Design review of the part built by this model. Coordinates are the model's own, in mm. Face numbers are marked on the shaded views. A direction names the side the tool comes from. Round coordinates to 2 decimals unless told otherwise and drop trailing zeros. Loops run counter-clockwise (first coordinate to the right, second up) from the corner with the lowest first, then second, coordinate; pieces in that order, holes last. Notation, with made-up numbers: (88.5, 50.25) - (124.5, 50.25) arc R27 cw to (124.5, 87.25) - close; hole circle Ø2 at (26.25, -24). An arc over 180 degrees is marked (long way). Return JSON: item names as keys, results as strings. Group by question number.
(1) We need section D-D, the plane z = -5.5. Write out the cut boundary in (x, y), and give its area (3 significant figures).
(2) We need section B-B, the plane y = 75. Write out the cut boundary in (x, z) (3 decimals).
(3) We need section C-C, the plane y = 45.5. Write out the cut boundary in (x, z).
(4) We need section A-A, the plane y = 7. Write out the cut boundary in (x, z), and give its area (3 significant figures).
(5) Wall thickness on L1, parallel to Z at x = 18.7, y = 75 (3 decimals); L2, parallel to Y at x = 17, z = -60.5; L3, parallel to Y at x = 10, z = -48.2: over which ranges is each line inside the solid? List them lowest first. Write a range as [from, to].
(6) Clearance check with flat-ended pins moving along their axes: pin 1 (4.5 mm diameter, centred on x = 10, y = -7, fed in from -Z); pin 2 (2 mm diameter, centred on y = 85, z = 1.175, fed in from -X); pin 3 (10 mm diameter, centred on x = 10.5, z = -7.5, fed in from -Y); pin 4 (6 mm diameter, centred on x = 11.5, y = 5, fed in from +Z). State where each tip first meets the part, or that it passes through.
(7) The part is to be moulded in two halves that separate along Z. For the marked faces 1, 2, 3 and 4, say which applies: pulls with the +Z half, pulls with the -Z half, needs draft (parallel to the pull), parting line crosses it, or undercut.
(8) For the marked faces 5, 6, 7, 8 and 9, list the 3-axis set-ups (+Z, -Z, +X, -X, +Y, -Y) from which the entire face can be reached by the end or side of a thin tool; tool diameter is ignored.
from build123d import *

# Parameters (mm, degrees)
EXTRUDE_1_DEPTH     = 2
SKETCH_2_R          = 1.65
CUT_EXTRUDE_1_DEPTH = 2
SKETCH_3_W          = 20
SKETCH_3_H          = 2
EXTRUDE_2_DEPTH     = 30
SKETCH_4_W          = 20
SKETCH_4_H          = 2
EXTRUDE_3_DEPTH     = 80
SKETCH_5_W          = 20
SKETCH_5_H          = 2
EXTRUDE_4_DEPTH     = 109.65
SKETCH_6_W          = 20
SKETCH_6_H          = 2
EXTRUDE_5_DEPTH     = 80
CUT_EXTRUDE_2_REACH = 126.622
SKETCH_8_R          = 3
SKETCH_9_W          = 2
SKETCH_9_H          = 5
EXTRUDE_6_DEPTH     = 20
SKETCH_10_R         = 1.65
CUT_EXTRUDE_3_DEPTH = 20
SKETCH_11_R         = 3.3
CUT_EXTRUDE_4_DEPTH = 10
SKETCH_12_W         = 45
SKETCH_12_H         = 2
EXTRUDE_7_DEPTH     = 14
SKETCH_13_W         = 2
SKETCH_13_H         = 45
EXTRUDE_8_DEPTH     = 20
SKETCH_14_R         = 3
CUT_EXTRUDE_6_DEPTH = 20


with BuildPart() as part:
    # 草图1 → 凸台-拉伸1 (new body)
    with BuildSketch(Plane.XY):
        with BuildLine():
            Line((0, 0), (0, 12))
            Line((0, 12), (20, 12))
            Line((20, 12), (20, 0))
            ThreePointArc((20, 0), (10, -10), (0, 0))
        make_face()
    extrude_1 = extrude(amount=EXTRUDE_1_DEPTH)

    # 草图2 → 切除-拉伸1 (cut)
    with BuildSketch(Plane.XY.offset(2)):
        with Locations((17, 0)):
            Circle(SKETCH_2_R)
        with Locations((10, -7)):
            Circle(SKETCH_2_R)
        with Locations((3, 0)):
            Circle(SKETCH_2_R)
        with Locations((10, 7)):
            Circle(SKETCH_2_R)
    extrude(amount=-CUT_EXTRUDE_1_DEPTH, mode=Mode.SUBTRACT)

    # 草图3 → 凸台-拉伸2 (add)
    with BuildSketch(Plane.XY.offset(2)):
        with Locations((10, 11)):
            Rectangle(SKETCH_3_W, SKETCH_3_H)
    extrude_2 = extrude(amount=EXTRUDE_2_DEPTH)

    # 草图4 → 凸台-拉伸3 (add)
    with BuildSketch(Plane(origin=(0, 12, 0), x_dir=(1, 0, 0), z_dir=(0, 1, 0))):
        with Locations((10, -31)):
            Rectangle(SKETCH_4_W, SKETCH_4_H)
    extrude(amount=EXTRUDE_3_DEPTH)

    # 草图5 → 凸台-拉伸4 (add)
    with BuildSketch(Plane(origin=(0, 0, 30), x_dir=(-1, 0, 0), z_dir=(0, 0, -1))):
        with Locations((-10, 91)):
            Rectangle(SKETCH_5_W, SKETCH_5_H)
    extrude(amount=EXTRUDE_4_DEPTH)

    # 草图6 → 凸台-拉伸5 (add)
    with BuildSketch(Plane.XZ.offset(-90)):
        with Locations((10, -78.65)):
            Rectangle(SKETCH_6_W, SKETCH_6_H)
    extrude(amount=EXTRUDE_5_DEPTH)

    # 镜向2: 凸台-拉伸2 across plane
    add(extrude_2.mirror(Plane.XY.offset(-23.825)))

    # 镜向3: 凸台-拉伸1 across plane
    add(extrude_1.mirror(Plane.XY.offset(-23.825)))

    # 草图8 → 切除-拉伸2 (cut, up to next)
    with BuildSketch(Plane(origin=(0, 0, -49.65), x_dir=(-1, 0, 0), z_dir=(0, 0, -1)), mode=Mode.PRIVATE) as cut_extrude_2_sk1:
        with Locations((-10, 0)):
            Circle(SKETCH_8_R)
    cut_extrude_2_tool1 = extrude(cut_extrude_2_sk1.sketch, amount=-CUT_EXTRUDE_2_REACH, mode=Mode.PRIVATE) & part.part
    add(cut_extrude_2_tool1.solids().sort_by_distance((10, 0, -49.65))[0], mode=Mode.SUBTRACT)

    # 草图9 → 凸台-拉伸6 (add)
    with BuildSketch(Plane.XZ.offset(-90)):
        with Locations((19, 1.175)):
            Rectangle(SKETCH_9_W, SKETCH_9_H)
        with Locations((19, -48.825)):
            Rectangle(SKETCH_9_W, SKETCH_9_H)
    extrude(amount=EXTRUDE_6_DEPTH)

    # 草图10 → 切除-拉伸3 (cut)
    with BuildSketch(Plane(origin=(20, 0, 0), x_dir=(0, 0, -1), z_dir=(1, 0, 0))):
        with Locations((-1.175, 75)):
            Circle(SKETCH_10_R)
        with Locations((-1.175, 85)):
            Circle(SKETCH_10_R)
        with Locations((48.825, 75)):
            Circle(SKETCH_10_R)
        with Locations((48.825, 85)):
            Circle(SKETCH_10_R)
    extrude(amount=-CUT_EXTRUDE_3_DEPTH, mode=Mode.SUBTRACT)

    # 草图11 → 切除-拉伸4 (cut)
    with BuildSketch(Plane(origin=(0, 92, 0), x_dir=(1, 0, 0), z_dir=(0, 1, 0))):
        with Locations(Location((10, 63.825, 0), (0, 0, 270))):
            Circle(SKETCH_11_R)
        with Locations(Location((10, -16.175, 0), (0, 0, 270))):
            Circle(SKETCH_11_R)
    extrude(amount=-CUT_EXTRUDE_4_DEPTH, mode=Mode.SUBTRACT)

    # 草图12 → 凸台-拉伸7 (add)
    with BuildSketch(Plane.ZY):
        with Locations((-23.825, 91)):
            Rectangle(SKETCH_12_W, SKETCH_12_H)
    extrude(amount=EXTRUDE_7_DEPTH)

    # 草图13 → 凸台-拉伸8 (add)
    with BuildSketch(Plane.XZ.offset(-90)):
        with Locations((-13, -23.825)):
            Rectangle(SKETCH_13_W, SKETCH_13_H)
    extrude(amount=EXTRUDE_8_DEPTH)

    # 草图14 → 切除-拉伸6 (cut)
    with BuildSketch(Plane.ZY.offset(14)):
        with Locations((-12.725, 80)):
            Circle(SKETCH_14_R)
    extrude(amount=-CUT_EXTRUDE_6_DEPTH, mode=Mode.SUBTRACT)


solid = part.part
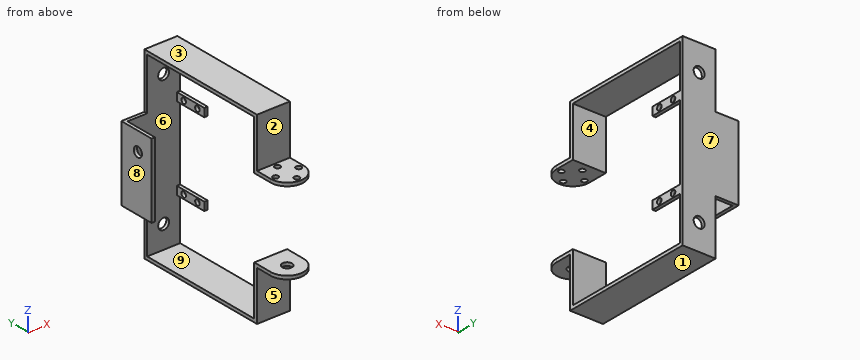
Solutions:
{
 "1": {"outline": "(-14, 70) - (-12, 70) - (-12, 90) - (20, 90) - (20, 92) - (-14, 92) - close", "area": "108 mm^2"},
 "2": {"outline": "(-14, -46.325) - (-12, -46.325) - (-12, -1.325) - (-14, -1.325) - close; (0, -79.65) - (20, -79.65) - (20, -77.65) - (0, -77.65) - close; (0, 30) - (20, 30) - (20, 32) - (0, 32) - close; (18, -51.325) - (20, -51.325) - (20, -50.475) - (18, -50.475) - close; (18, -47.175) - (20, -47.175) - (20, -46.325) - (18, -46.325) - close; (18, -1.325) - (20, -1.325) - (20, -0.475) - (18, -0.475) - close; (18, 2.825) - (20, 2.825) - (20, 3.675) - (18, 3.675) - close"},
 "3": {"outline": "(0, -79.65) - (20, -79.65) - (20, -77.65) - (0, -77.65) - close; (0, 30) - (20, 30) - (20, 32) - (0, 32) - close"},
 "4": {"outline": "(0, -49.65) - (20, -49.65) - (20, -47.65) - (0, -47.65) - close; (0, 0) - (8.35, 0) - (8.35, 2) - (0, 2) - close; (11.65, 0) - (20, 0) - (20, 2) - (11.65, 2) - close", "area": "73.4 mm^2"},
 "5": {"L1": "[-79.65, -77.65], [-51.325, -50.475], [-47.175, -46.325], [-1.325, -0.475], [2.825, 3.675], [30, 32]", "L2": "[10, 12], [90, 92]", "L3": "[-10, -3], [3, 12], [90, 92]"},
 "6": {"pin 1": "z = -49.65", "pin 2": "through", "pin 3": "y = 90", "pin 4": "z = 2"},
 "7": {"face 1": "pulls with the -Z half", "face 2": "needs draft", "face 3": "pulls with the +Z half", "face 4": "undercut"},
 "8": {"face 5": "-Z, +X, -X, -Y", "face 6": "none", "face 7": "+Z, -Z, +X, -X, +Y", "face 8": "+Z, -Z, -X, +Y, -Y", "face 9": "+X, -X"}
}
